Could you check a few things on this model? Use its own coordinates, in mm. A direction names the side the tool comes from. Give positions to 0.01 mm unless a question says otherwise; leave off trailing zeros. Loops run counter-clockwise (first coordinate to the right, second up) from the corner with the lowest first, then second, coordinate; pieces in that order, holes last. Notation, with made-up numbers: M -10,51 L 0,51 A22 ccw 0,71 Z; hole C 81,3 d8. An arc over 180 degrees is marked long. Return JSON: item names as keys, results as strings. Group by question number.
1. If we mould it in two halves opening along Y, with no side actions, what happens to faces 1 (the cylindrical face through (-27.1, -23.9, 14.2)), 2 (the flat face through (31, 0, 16.51)), 3 (the cylindrical face through (36.93, -13.463, 14.006)), 4 (the flat face through (0, -22.86, 15))? For each: +Y half, -Y half, draft (parallel to the pull), parting line (faces both ways), or undercut.
2. Please list where these lines run through material, in increasing order: line 1 (X direction, y = 20.5, z = 24); line 2 (Y direction, x = 13.5, z = 5); line 3 (X direction, y = 4.5, z = 11.5) (3 decimals).
3. For pin 1 (3 mm diameter, centred on x = -14.5, y = -14, fed in from +Z); pin 2 (3.5 mm diameter, centred on y = -10, z = 24.5, fed in from +X) (3 decimals); pin 3 (8 mm diameter, centred on x = 34, y = -11, fed in from -Z), each with a flat end and sliding along its axis, tell me the tip position at first contact or that it passes through.
4. If we section it at D-D (y = -16): Write out the boundary of the cut face in (x, z) (3 decimals), plus the area to 3 significant figures.
5. For faces 5 (the cylindrical face through (32.92, 13.463, 14.006)), 6 (the flat face through (28.575, 0, 22)), 7 (the cylindrical face through (25.271, -22.136, 15.418)), 8 (the cylindrical face through (27.05, -23.95, 22.31)), which set-ups out of +Z, -Z, +X, -X, +Y, -Y let a thin tool reach every point of the face, with its end or its side?
6. If we section it at B-B (z = 6): Write out the boundary of the cut face in (x, y) (3 decimals).
7. If we section it at A-A (y = 0): Write out the boundary of the cut face in (x, z) (1 decimal), plus the area to 3 significant figures.
8. If we section it at C-C (x = -10): Write out the boundary of the cut face in (y, z).
```python
from build123d import *

# Parameters (mm, degrees)
F0_W      = 57.15
F0_H      = 50.8
F1_DEPTH  = 27.94
F2_R      = 5.08
F5_DEPTH  = 2.54
F7_DEPTH  = 25.4
F9_DEPTH  = 2.54
F10_R     = 3.175
F11_DEPTH = 50.801
F13_DEPTH = 5.08


with BuildPart() as f1:
    # F0 (on Top) → F1 (new body)
    with BuildSketch(Plane.XY):
        Rectangle(F0_W, F0_H)
    extrude(amount=F1_DEPTH)

    # F2
    f2_edges = [f1.edges().sort_by_distance(p)[0] for p in [
        (-28.575, 25.4, 13.97),
        (28.575, 25.4, 13.97),
        (28.575, -25.4, 13.97),
        (-28.575, -25.4, 13.97),
    ]]
    fillet(f2_edges, radius=F2_R)

    # F4 (on offset) → F5 (join, symmetric)
    with BuildSketch(Plane(origin=(0, 0, 13.97), x_dir=(1, 0, 0), z_dir=(0, 0, -1))):
        with BuildLine():
            Line((36.195, 25.4), (23.495, 25.4))
            Line((23.495, 25.4), (23.495, -25.4))
            Line((23.495, -25.4), (36.195, -25.4))
            ThreePointArc((36.195, -25.4), (40.685128, -23.540128), (42.545, -19.05))
            Line((42.545, -19.05), (42.545, 19.05))
            ThreePointArc((42.545, 19.05), (40.685128, 23.540128), (36.195, 25.4))
        make_face()
    extrude(amount=F5_DEPTH, both=True)

    # F6 (on face) → F7 (cut)
    with BuildSketch(Plane.XY.offset(27.94)):
        with BuildLine():
            ThreePointArc((-26.035, -20.32), (-25.291051, -22.116051), (-23.495, -22.86))
            Line((-23.495, -22.86), (23.495, -22.86))
            ThreePointArc((23.495, -22.86), (25.291051, -22.116051), (26.035, -20.32))
            Line((26.035, -20.32), (26.035, 20.32))
            ThreePointArc((26.035, 20.32), (25.291051, 22.116051), (23.495, 22.86))
            Line((23.495, 22.86), (-23.495, 22.86))
            ThreePointArc((-23.495, 22.86), (-25.291051, 22.116051), (-26.035, 20.32))
            Line((-26.035, 20.32), (-26.035, -20.32))
        make_face()
    extrude(amount=-F7_DEPTH, mode=Mode.SUBTRACT)

    # F8 (on face) → F9 (cut, through all)
    with BuildSketch(Plane(origin=(-28.575, 0, 0), x_dir=(0, -1, 0), z_dir=(-1, 0, 0))):
        with BuildLine():
            Line((3.398882, 20.828), (-3.398882, 20.828))
            ThreePointArc((-3.398882, 20.828), (0, 8.6995), (3.398882, 20.828))
        make_face()
    extrude(amount=-F9_DEPTH, mode=Mode.SUBTRACT)

    # F10 (on face) → F11 (cut, through all)
    with BuildSketch(Plane.XZ.offset(25.4)):
        with Locations((15.875, 13.97)):
            Circle(F10_R)
    extrude(amount=-F11_DEPTH, mode=Mode.SUBTRACT)

    # F12 (on face) → F13 (cut, through all)
    with BuildSketch(Plane.XY.offset(16.51)):
        with BuildLine():
            Line((35.687, 13.97), (34.163, 13.97))
            ThreePointArc((34.163, 13.97), (32.905764, 13.449236), (32.385, 12.192))
            Line((32.385, 12.192), (32.385, -12.192))
            ThreePointArc((32.385, -12.192), (32.905764, -13.449236), (34.163, -13.97))
            Line((34.163, -13.97), (35.687, -13.97))
            ThreePointArc((35.687, -13.97), (36.944236, -13.449236), (37.465, -12.192))
            Line((37.465, -12.192), (37.465, 12.192))
            ThreePointArc((37.465, 12.192), (36.944236, 13.449236), (35.687, 13.97))
        make_face()
    extrude(amount=-F13_DEPTH, mode=Mode.SUBTRACT)


solid = f1.part
```
Answer:
{
 "1": {"face 1": "-Y half", "face 2": "draft", "face 3": "undercut", "face 4": "undercut"},
 "2": {"line 1": "x = -28.57 to -26.03, 26.03 to 28.57", "line 2": "y = -25.4 to -22.86, 22.86 to 25.4", "line 3": "x = 26.035 to 32.385, 37.465 to 42.545"},
 "3": {"pin 1": "stops at z = 2.54", "pin 2": "stops at x = 28.575", "pin 3": "stops at z = 11.43"},
 "4": {"outline": "M -28.575,0 L 28.575,0 L 28.575,11.43 L 42.545,11.43 L 42.545,16.51 L 28.575,16.51 L 28.575,27.94 L 26.035,27.94 L 26.035,2.54 L -26.035,2.54 L -26.035,27.94 L -28.575,27.94 Z", "area": "345 mm²"},
 "5": {"face 5": "+Z, -Z", "face 6": "+Z, +X, +Y, -Y", "face 7": "+Z", "face 8": "+Z, +X, -Y"},
 "6": {"outline": "M -28.575,-20.32 A5.08 ccw -23.495,-25.4 L 23.495,-25.4 A5.08 ccw 28.575,-20.32 L 28.575,20.32 A5.08 ccw 23.495,25.4 L -23.495,25.4 A5.08 ccw -28.575,20.32 Z; hole M -26.035,-20.32 A2.54 ccw -23.495,-22.86 L 23.495,-22.86 A2.54 ccw 26.035,-20.32 L 26.035,20.32 A2.54 ccw 23.495,22.86 L -23.495,22.86 A2.54 ccw -26.035,20.32 Z"},
 "7": {"outline": "M -28.6,0 L 28.6,0 L 28.6,11.4 L 32.4,11.4 L 32.4,16.5 L 28.6,16.5 L 28.6,27.9 L 26,27.9 L 26,2.5 L -26,2.5 L -26,8.7 L -28.6,8.7 Z; M -28.6,20.8 L -26,20.8 L -26,27.9 L -28.6,27.9 Z; M 37.5,11.4 L 42.5,11.4 L 42.5,16.5 L 37.5,16.5 Z", "area": "289 mm²"},
 "8": {"outline": "M -25.4,0 L 25.4,0 L 25.4,27.94 L 22.86,27.94 L 22.86,2.54 L -22.86,2.54 L -22.86,27.94 L -25.4,27.94 Z"}
}
